```python
from build123d import *

# Parameters (mm, degrees)
SKETCH2_W            = 68.58
SKETCH2_H            = 76.2
BOSS_EXTRUDE1_DEPTH  = 1.5875
M4_CLEARANCE_HOLE1_D = 4.8
SKETCH5_R            = 15
CUT_EXTRUDE1_DEPTH   = 52.356545104
BOSS_EXTRUDE2_DEPTH  = 3.175


with BuildPart() as part:
    # Sketch2 → Boss-Extrude1 (new, symmetric)
    with BuildSketch(Plane.XY):
        Rectangle(SKETCH2_W, SKETCH2_H)
    extrude(amount=BOSS_EXTRUDE1_DEPTH, both=True)

    # M4 Clearance Hole1 (through all)
    with Locations(Plane.XY.offset(1.5875)):
        with Locations((-23.368, -19.558), (-23.368, 31.242), (27.432, 31.242), (27.432, -19.558)):
            Hole(M4_CLEARANCE_HOLE1_D / 2)

    # Sketch5 → Cut-Extrude1 (cut, through all)
    with BuildSketch(Plane.XY.offset(1.5875)):
        with Locations((1.884, 5.842)):
            Circle(SKETCH5_R)
    extrude(amount=-CUT_EXTRUDE1_DEPTH, mode=Mode.SUBTRACT)

    # Sketch6 → Boss-Extrude2 (add, through all)
    with BuildSketch(Plane(origin=(0, 0, -1.5875), x_dir=(-1, 0, 0), z_dir=(0, 0, -1))):
        Polygon((-39.37, 43.18), (-39.37, -38.1), (-34.29, -38.1), (-34.29, 38.1), (34.29, 38.1), (34.29, -38.1), (39.37, -38.1), (39.37, 43.18), align=None)
    extrude(amount=-BOSS_EXTRUDE2_DEPTH)


solid = part.part
```
Read the model definition and answer for the solid it produces. Units are mm, in the model's axes. Coordinates: 2 decimals unless noted, no trailing zeros. Write each loop counter-clockwise with the first axis right and the second up, starting at its lowest first coordinate (ties: lowest second). Pieces come first, ordered by that corner, then holes. Notation, with made-up numbers: (33, 7.25) -> (75, 7.25) arc R35 cw to (75, 42.25) -> close; hole circle Ø9 at (72, 86.25). An arc over 180 degrees is marked (long way). Return JSON: item names as keys, results as strings.
1. A cutting plane is placed at B-B (y = 14). Determine the outline of the cut face in (x, z), and give its area (3 significant figures).
Found:
{"outline": "(-39.37, -1.59) -> (-10.7, -1.59) -> (-10.7, 1.59) -> (-39.37, 1.59) -> close; (14.47, -1.59) -> (39.37, -1.59) -> (39.37, 1.59) -> (14.47, 1.59) -> close", "area": "170 mm2"}
2. Find the intervals of material crossed by line 1 along X through (y, z) = (-18, 0.7); line 2 along X through (y, z) = (1, -0.25); line 3 along Y through (x, z) = (3, 0.55), in increasing order. Write a range as from..to.
Found:
{"line 1": "-39.37..-25.19, -21.54..25.61, 29.26..39.37", "line 2": "-39.37..-12.31, 16.08..39.37", "line 3": "-38.1..-9.12, 20.8..43.18"}
3. This flat-tipped pin is pushed along its axis until it touches: P1, Ø4.5, axis at x = -23.368, y = 31.242, coming from the -Z side. Where does it stop, or does it pass through?
Found:
{"P1": "through"}
4. A cutting plane is placed at C-C (z = 0.5). Determine the outline of the cut face in (x, y).
Found:
{"outline": "(-39.37, -38.1) -> (39.37, -38.1) -> (39.37, 43.18) -> (-39.37, 43.18) -> close; hole circle Ø4.8 at (-23.37, -19.56); hole circle Ø4.8 at (-23.37, 31.24); hole circle Ø30 at (1.88, 5.84); hole circle Ø4.8 at (27.43, -19.56); hole circle Ø4.8 at (27.43, 31.24)"}
5. A cutting plane is placed at A-A (x = 2.5). Determine the outline of the cut face in (y, z).
Found:
{"outline": "(-38.1, -1.59) -> (-9.15, -1.59) -> (-9.15, 1.59) -> (-38.1, 1.59) -> close; (20.83, -1.59) -> (43.18, -1.59) -> (43.18, 1.59) -> (20.83, 1.59) -> close"}
6. Determine the mould class of faces 1 (the face through (-25, 33, 0)), 2 (the face through (-8, -6, -1.588)), 3 (the face through (1, -38.1, 0)) for opening direction Y: pulls with the +Y half, pulls with the -Y half, needs draft (parallel to the pull), parting line crosses it, or undercut.
Found:
{"face 1": "undercut", "face 2": "needs draft", "face 3": "pulls with the -Y half"}
